from build123d import *

# Parameters (mm, degrees)
SKETCH_1_R           = 20
SKETCH_1_R_2         = 16
EXTRUDE_1_DEPTH      = 40
SKETCH_2_R           = 20
EXTRUDE_2_DEPTH      = 4
SKETCH_3_R           = 3
CUT_EXTRUDE_1_DEPTH  = 4
CUT_EXTRUDE_2_DEPTH  = 2
EXTRUDE_START        = 4
SKETCH_7_R           = 20
EXTRUDE_3_DEPTH      = 4
SKETCH_8_R           = 1.5
CUT_EXTRUDE_4_DEPTH  = 6
SKETCH_10_W          = 10
SKETCH_10_H          = 30
CUT_EXTRUDE_6_DEPTH  = 48
SKETCH_11_W          = 22.45751311
SKETCH_11_H          = 40
CUT_EXTRUDE_9_DEPTH  = 25
CUT_EXTRUDE_10_DEPTH = 2
SKETCH_14_R          = 2
CUT_EXTRUDE_11_DEPTH = 4
CUT_EXTRUDE_12_DEPTH = 2
SKETCH_16_R          = 0.5
CUT_EXTRUDE_13_DEPTH = 55


with BuildPart() as part:
    # 草图1 → 凸台-拉伸1 (new body)
    with BuildSketch(Plane(origin=(0, 0, 0), x_dir=(1, 0, 0), z_dir=(0, 1, 0))):
        with Locations(Location((0, 0, 0), (0, 0, 270))):
            Circle(SKETCH_1_R)
        with Locations(Location((0, 0, 0), (0, 0, 270))):
            Circle(SKETCH_1_R_2, mode=Mode.SUBTRACT)
    extrude(amount=EXTRUDE_1_DEPTH)

    # 草图2 → 凸台-拉伸2 (add)
    with BuildSketch(Plane(origin=(0, 40, 0), x_dir=(1, 0, 0), z_dir=(0, 1, 0))):
        with Locations(Location((0, 0, 0), (0, 0, 270))):
            Circle(SKETCH_2_R)
    extrude(amount=EXTRUDE_2_DEPTH)

    # 草图3 → 切除-拉伸1 (cut)
    with BuildSketch(Plane(origin=(0, 44, 0), x_dir=(1, 0, 0), z_dir=(0, 1, 0))):
        with Locations(Location((0, 0, 0), (0, 0, 270))):
            Circle(SKETCH_3_R)
    extrude(amount=-CUT_EXTRUDE_1_DEPTH, mode=Mode.SUBTRACT)

    # 草图5 → 切除-拉伸2 (cut)
    with BuildSketch(Plane.XZ.offset(-40)):
        with BuildLine():
            Line((3, 10), (3, -10))
            ThreePointArc((3, -10), (0, -13), (-3, -10))
            Line((-3, -10), (-3, 10))
            ThreePointArc((-3, 10), (0, 13), (3, 10))
        make_face()
    extrude(amount=-CUT_EXTRUDE_2_DEPTH, mode=Mode.SUBTRACT)

    # 草图7 → 凸台-拉伸3 (add)
    with BuildSketch(Plane.XZ.offset(EXTRUDE_START)):
        with Locations(Location((0, 0, 0), (0, 0, 270))):
            Circle(SKETCH_7_R)
    extrude(amount=-EXTRUDE_3_DEPTH)

    # 草图8 → 切除-拉伸4 (cut)
    with BuildSketch(Plane.XZ.offset(4)):
        with Locations(Location((0, 0, 0), (0, 0, 270))):
            Circle(SKETCH_8_R)
    extrude(amount=-CUT_EXTRUDE_4_DEPTH, mode=Mode.SUBTRACT)

    # 草图10 → 切除-拉伸6 (cut)
    with BuildSketch(Plane(origin=(0, 44, 0), x_dir=(1, 0, 0), z_dir=(0, 1, 0))):
        with Locations((-20, 0)):
            Rectangle(SKETCH_10_W, SKETCH_10_H)
    extrude(amount=-CUT_EXTRUDE_6_DEPTH, mode=Mode.SUBTRACT)

    # 草图11 → 切除-拉伸9 (cut)
    with BuildSketch(Plane.ZY.offset(15)):
        with Locations((0, 20)):
            Rectangle(SKETCH_11_W, SKETCH_11_H)
    extrude(amount=-CUT_EXTRUDE_9_DEPTH, mode=Mode.SUBTRACT)

    # 草图12 → 切除-拉伸10 (cut)
    with BuildSketch(Plane(origin=(0, 0, 0), x_dir=(1, 0, 0), z_dir=(0, 1, 0))):
        Polygon((0, 2.886751346), (-2.5, 1.443375673), (-2.5, -1.443375673), (0, -2.886751346), (2.5, -1.443375673), (2.5, 1.443375673), align=None)
    extrude(amount=-CUT_EXTRUDE_10_DEPTH, mode=Mode.SUBTRACT)

    # 草图14 → 切除-拉伸11 (cut)
    with BuildSketch(Plane.XZ.offset(-40)):
        with Locations(Location((10.674541512, 0, 0), (0, 0, 270))):
            Circle(SKETCH_14_R)
    extrude(amount=-CUT_EXTRUDE_11_DEPTH, mode=Mode.SUBTRACT)

    # 草图15 → 切除-拉伸12 (cut)
    with BuildSketch(Plane.XZ.offset(-40)):
        with BuildLine():
            Line((-7, 3), (5.528448646, 3))
            ThreePointArc((5.528448646, 3), (8.528448646, 0), (5.528448646, -3))
            Line((5.528448646, -3), (-7, -3))
            ThreePointArc((-7, -3), (-10, 0), (-7, 3))
        make_face()
    extrude(amount=-CUT_EXTRUDE_12_DEPTH, mode=Mode.SUBTRACT)

    # 草图16 → 切除-拉伸13 (cut, through all)
    with BuildSketch(Plane.XZ.offset(-42)):
        with Locations(Location((0, 12, 0), (0, 0, 270))):
            Circle(SKETCH_16_R)
        with Locations(Location((0, 10, 0), (0, 0, 270))):
            Circle(SKETCH_16_R)
        with Locations(Location((0, 8, 0), (0, 0, 270))):
            Circle(SKETCH_16_R)
        with Locations(Location((0, 6, 0), (0, 0, 270))):
            Circle(SKETCH_16_R)
        with Locations(Location((-7.531348858, 0, 0), (0, 0, 270))):
            Circle(SKETCH_16_R)
        with Locations(Location((-5.531348858, 0, 0), (0, 0, 270))):
            Circle(SKETCH_16_R)
        with Locations(Location((5.531348858, 0, 0), (0, 0, 90))):
            Circle(SKETCH_16_R)
        with Locations(Location((7.531348858, 0, 0), (0, 0, 90))):
            Circle(SKETCH_16_R)
        with Locations(Location((0, -6, 0), (0, 0, 90))):
            Circle(SKETCH_16_R)
        with Locations(Location((0, -8, 0), (0, 0, 90))):
            Circle(SKETCH_16_R)
        with Locations(Location((0, -10, 0), (0, 0, 90))):
            Circle(SKETCH_16_R)
        with Locations(Location((0, -12, 0), (0, 0, 90))):
            Circle(SKETCH_16_R)
    extrude(amount=-CUT_EXTRUDE_13_DEPTH, mode=Mode.SUBTRACT)


solid = part.part
Read the model definition and answer for the solid it produces. Units are mm, in the model's axes. A direction names the side the tool comes from. Round coordinates to 2 decimals unless told otherwise and drop trailing zeros. Loops run counter-clockwise (first coordinate to the right, second up) from the corner with the lowest first, then second, coordinate; pieces in that order, holes last. Notation, with made-up numbers: (-26.75, 58) - (-14.75, 58) arc R9 cw to (-14.75, 75) - close; hole circle Ø11 at (15, 1). An arc over 180 degrees is marked (long way). One line per question, with ' | ' between items. Start each with the question number.
Q1. Section B-B on y = 28.5 is taken. Give the vertices of the cut face in (x, z).
Q2. Find the intervals of material crossed by L1, parallel to Y at x = 12, z = -3.5; L2, parallel to X at y = 15, z = 13.5; L3, parallel to Y at x = 5, z = 1, in increasing order.
Q3. Flat-ended cylindrical pins translate along their axes: pin 1 (1.6 mm diameter, centred on x = -6, y = 41.5, fed in from +Z); pin 2 (1.6 mm diameter, centred on x = -5.5, y = 41.5, fed in from -Z); pin 3 (1 mm diameter, centred on y = 35.5, z = 1.5, fed in from -X). Find the tip coordinate at first contact, or state that the pin passes through.
Q4. For a pull along Z with two mould halves and no side action, classify faces 1 (the flat face through (3, -4, 0)), 2 (the cylindrical face through (19.99, 19.66, -0.68)), 3 (the flat face through (4, 41, 3)) as +Z half, -Z half, draft (parallel to the pull), parting line (faces both ways), or undercut.
Q5. For faces 4 (the flat face through (-15, 20, 12)), 5 (the flat face through (1.267, -0.986, -2.155)), 6 (the flat face through (-13, 20, -11.229)), 7 (the flat face through (-3, 41, -7)), determine the directions among +Z, -Z, +X, -X, +Y, -Y from which every point of the face is accessible in a straight line to the end or side of a thin tool.
Q6. Section A-A on y = 41 is taken. Give the vertices of the cut face in (x, z), plus the area to 3 significant figures.
Established:
1) outline: (-15, -13.23) arc R20 ccw (long way) to (-15, 13.23) - (-15, 11.23) - (-11.4, 11.23) arc R16 cw (long way) to (-11.4, -11.23) - (-15, -11.23) - close
2) L1: -4 to 0, 40 to 44 | L2: -14.76 to -8.59, 8.59 to 14.76 | L3: -4 to 0, 42 to 44
3) pin 1: z = 19.31 | pin 2: z = -19.44 | pin 3: x = 15.87
4) face 1: draft | face 2: parting line | face 3: undercut
5) face 4: +Z, -Z, -X, +Y, -Y | face 5: +Y | face 6: -X | face 7: none
6) outline: (-15, -13.23) arc R20 ccw (long way) to (-15, 13.23) - close; hole (-7, -3) - (-3, -3) - (-3, -10) arc R3 ccw to (3, -10) - (3, -3) - (5.53, -3) arc R3 ccw to (5.53, 3) - (3, 3) - (3, 10) arc R3 ccw to (-3, 10) - (-3, 3) - (-7, 3) arc R3 ccw to start; hole circle Ø4 at (10.67, 0) | area: 938 mm²
